Check sheet for the modelled part. Datum: model origin and axes. Units: mm. A direction names the side the tool comes from. Round coordinates to 2 decimals unless told otherwise and drop trailing zeros. Loops run counter-clockwise (first coordinate to the right, second up) from the corner with the lowest first, then second, coordinate; pieces in that order, holes last. Notation, with made-up numbers: M 67.5,-5.5 L 97.5,-5.5 A17 ccw 97.5,27.5 Z; hole C 39,-36.5 d1. An arc over 180 degrees is marked long. Write item = value, one per line. Start each with the question number.
(1) Set-up check for faces 1 (the face through (-38, -3, -9.525)), 2 (the face through (76.2, -3, -1)): record each of +Z, -Z, +X, -X, +Y, -Y from which the full face is reachable in a straight line by a thin tool's end or side.
(2) Go/stop test with flat-tipped pins: P1, Ø8, axis at x = 36.5, z = 8.5, coming from the +Y side; P2, Ø11.5, axis at x = 38.1, z = -30.48, coming from the +Y side. Record where each tip stops, or that it passes through.
(3) Mould release check, pull along Z, two halves, no side actions. Record for faces 3 (the face through (-72.58, -3.22, -53.33)), 4 (the face through (72.58, -3.22, 53.33)), 5 (the face through (-38, -3, -3.175)): pulls with the +Z half, pulls with the -Z half, needs draft (parallel to the pull), parting line crosses it, or undercut.
(4) Cross-section at A-A on x = 38.1. Record the boundary of the cut face in (y, z) (3 decimals).
(5) Scan lines: L1, parallel to Z at x = 38.1, y = -4 (3 decimals); L2, parallel to Z at x = 33, y = -3.75; L3, parallel to X at y = -4.25, z = 29. Record each from-to range of solid material in increasing order. Write a range as from..to.
(6) Cross-section at C-C on x = -27.5. State how many separate pieces and enclosed holes the cut face has, plus the area to 3 significant figures.
(7) Cross-section at B-B on z = 0. Record the boundary of the cut face in (x, y) (3 decimals), plus the area to 3 significant figures.
from build123d import *

# Parameters (mm, degrees)
F0_W         = 152.4
F0_H         = 114.3
F1_DEPTH     = 6.35
F2_R         = 12.7
F3_R         = 9.525
F4_DEPTH     = 25.4
F5_R         = 9.525
F6_DEPTH     = 25.4
F7_R         = 9.525
F8_DEPTH     = 25.4
F16_W        = 50.8
F16_H        = 6.35
F15_W        = 50.8
F15_H        = 6.35
F14_W        = 50.8
F14_H        = 6.35
F13_W        = 50.8
F13_H        = 6.35
F12_W        = 50.8
F12_H        = 6.35
F11_W        = 50.8
F11_H        = 6.35
F10_W        = 50.8
F10_H        = 6.35
F9_W         = 50.8
F9_H         = 6.35
F17_DEPTH    = 25.4
F18_T1_DEPTH = 6.35
F19_T1_DEPTH = 6.35


# Not quite as in the source:
# - a fillet or chamfer that OpenCascade refuses, or shapes differently, is made with other operations: its cross-section is extruded or revolved along the edge and cut away or added


with BuildPart() as f1:
    # F0 (on Front) → F1 (new body)
    with BuildSketch(Plane.XZ):
        Rectangle(F0_W, F0_H)
    extrude(amount=F1_DEPTH)

    # F2
    f2_edges = [f1.edges().sort_by_distance(p)[0] for p in [
        (-76.2, -3.175, 57.15),
        (-76.2, -3.175, -57.15),
        (76.2, -3.175, -57.15),
        (76.2, -3.175, 57.15),
    ]]
    fillet(f2_edges, radius=F2_R)

    # F3 (on face) → F4 (cut)
    with BuildSketch(Plane.XZ.offset(6.35)):
        with Locations((38.1, 30.48)):
            Circle(F3_R)
    extrude(amount=-F4_DEPTH, mode=Mode.SUBTRACT)

    # F5 (on face) → F6 (cut)
    with BuildSketch(Plane.XZ.offset(6.35)):
        with Locations((38.1, 0)):
            Circle(F5_R)
    extrude(amount=-F6_DEPTH, mode=Mode.SUBTRACT)

    # F7 (on face) → F8 (cut)
    with BuildSketch(Plane.XZ.offset(6.35)):
        with Locations((38.1, -30.48)):
            Circle(F7_R)
    extrude(amount=-F8_DEPTH, mode=Mode.SUBTRACT)

    # F16 (on face) + F15 (on face) + F14 (on face) + F13 (on face) + F12 (on face) + F11 (on face) + F10 (on face) + F9 (on face) → F17 (cut)
    with BuildSketch(Plane.XZ.offset(6.35)):
        with Locations((-38.1, 44.45)):
            Rectangle(F16_W, F16_H)
    with BuildSketch(Plane.XZ.offset(6.35)):
        with Locations((-38.1, 31.75)):
            Rectangle(F15_W, F15_H)
    with BuildSketch(Plane.XZ.offset(6.35)):
        with Locations((-38.1, 19.05)):
            Rectangle(F14_W, F14_H)
    with BuildSketch(Plane.XZ.offset(6.35)):
        with Locations((-38.1, 6.35)):
            Rectangle(F13_W, F13_H)
    with BuildSketch(Plane.XZ.offset(6.35)):
        with Locations((-38.1, -6.35)):
            Rectangle(F12_W, F12_H)
    with BuildSketch(Plane.XZ.offset(6.35)):
        with Locations((-38.1, -19.05)):
            Rectangle(F11_W, F11_H)
    with BuildSketch(Plane.XZ.offset(6.35)):
        with Locations((-38.1, -31.75)):
            Rectangle(F10_W, F10_H)
    with BuildSketch(Plane.XZ.offset(6.35)):
        with Locations((-38.1, -44.45)):
            Rectangle(F9_W, F9_H)
    extrude(amount=-F17_DEPTH, mode=Mode.SUBTRACT)

    # F18: fillet of radius 3.81 on 16 edges, made by hand

    # F18_s2 → F18_t1 (join)
    with BuildSketch(Plane.XZ):
        with BuildLine():
            ThreePointArc((-12.7, 6.985), (-13.8159231637, 4.2909231637), (-16.51, 3.175))
            Line((-16.51, 3.175), (-12.7, 3.175))
            Line((-12.7, 3.175), (-12.7, 6.985))
        make_face()
        with BuildLine():
            ThreePointArc((-16.51, -9.525), (-13.8159231637, -8.4090768363), (-12.7, -5.715))
            Line((-12.7, -5.715), (-12.7, -9.525))
            Line((-12.7, -9.525), (-16.51, -9.525))
        make_face()
        with BuildLine():
            ThreePointArc((-12.7, -31.115), (-13.8159231637, -33.8090768363), (-16.51, -34.925))
            Line((-16.51, -34.925), (-12.7, -34.925))
            Line((-12.7, -34.925), (-12.7, -31.115))
        make_face()
        with BuildLine():
            ThreePointArc((-16.51, -22.225), (-13.8159231637, -21.1090768363), (-12.7, -18.415))
            Line((-12.7, -18.415), (-12.7, -22.225))
            Line((-12.7, -22.225), (-16.51, -22.225))
        make_face()
        with BuildLine():
            ThreePointArc((-12.7, -43.815), (-13.8159231637, -46.5090768363), (-16.51, -47.625))
            Line((-16.51, -47.625), (-12.7, -47.625))
            Line((-12.7, -47.625), (-12.7, -43.815))
        make_face()
        with BuildLine():
            ThreePointArc((-16.51, 15.875), (-13.8159231637, 16.9909231637), (-12.7, 19.685))
            Line((-12.7, 19.685), (-12.7, 15.875))
            Line((-12.7, 15.875), (-16.51, 15.875))
        make_face()
        with BuildLine():
            ThreePointArc((-16.51, 28.575), (-13.8159231637, 29.6909231637), (-12.7, 32.385))
            Line((-12.7, 32.385), (-12.7, 28.575))
            Line((-12.7, 28.575), (-16.51, 28.575))
        make_face()
        with BuildLine():
            ThreePointArc((-16.51, 41.275), (-13.8159231637, 42.3909231637), (-12.7, 45.085))
            Line((-12.7, 45.085), (-12.7, 41.275))
            Line((-12.7, 41.275), (-16.51, 41.275))
        make_face()
        with BuildLine():
            ThreePointArc((-12.7, -45.085), (-13.8159231637, -42.3909231637), (-16.51, -41.275))
            Line((-16.51, -41.275), (-12.7, -41.275))
            Line((-12.7, -41.275), (-12.7, -45.085))
        make_face()
        with BuildLine():
            ThreePointArc((-12.7, -32.385), (-13.8159231637, -29.6909231637), (-16.51, -28.575))
            Line((-16.51, -28.575), (-12.7, -28.575))
            Line((-12.7, -28.575), (-12.7, -32.385))
        make_face()
        with BuildLine():
            ThreePointArc((-12.7, -19.685), (-13.8159231637, -16.9909231637), (-16.51, -15.875))
            Line((-16.51, -15.875), (-12.7, -15.875))
            Line((-12.7, -15.875), (-12.7, -19.685))
        make_face()
        with BuildLine():
            ThreePointArc((-12.7, -6.985), (-13.8159231637, -4.2909231637), (-16.51, -3.175))
            Line((-16.51, -3.175), (-12.7, -3.175))
            Line((-12.7, -3.175), (-12.7, -6.985))
        make_face()
        with BuildLine():
            ThreePointArc((-12.7, 5.715), (-13.8159231637, 8.4090768363), (-16.51, 9.525))
            Line((-16.51, 9.525), (-12.7, 9.525))
            Line((-12.7, 9.525), (-12.7, 5.715))
        make_face()
        with BuildLine():
            ThreePointArc((-12.7, 18.415), (-13.8159231637, 21.1090768363), (-16.51, 22.225))
            Line((-16.51, 22.225), (-12.7, 22.225))
            Line((-12.7, 22.225), (-12.7, 18.415))
        make_face()
        with BuildLine():
            ThreePointArc((-12.7, 31.115), (-13.8159231637, 33.8090768363), (-16.51, 34.925))
            Line((-16.51, 34.925), (-12.7, 34.925))
            Line((-12.7, 34.925), (-12.7, 31.115))
        make_face()
        with BuildLine():
            ThreePointArc((-12.7, 43.815), (-13.8159231637, 46.5090768363), (-16.51, 47.625))
            Line((-16.51, 47.625), (-12.7, 47.625))
            Line((-12.7, 47.625), (-12.7, 43.815))
        make_face()
    extrude(amount=F18_T1_DEPTH)

    # F19: fillet of radius 3.81 on 16 edges, made by hand

    # F19_s2 → F19_t1 (join)
    with BuildSketch(Plane.XZ):
        with BuildLine():
            ThreePointArc((-59.69, 47.625), (-62.3840768363, 46.5090768363), (-63.5, 43.815))
            Line((-63.5, 43.815), (-63.5, 47.625))
            Line((-63.5, 47.625), (-59.69, 47.625))
        make_face()
        with BuildLine():
            ThreePointArc((-59.69, 34.925), (-62.3840768363, 33.8090768363), (-63.5, 31.115))
            Line((-63.5, 31.115), (-63.5, 34.925))
            Line((-63.5, 34.925), (-59.69, 34.925))
        make_face()
        with BuildLine():
            ThreePointArc((-59.69, 22.225), (-62.3840768363, 21.1090768363), (-63.5, 18.415))
            Line((-63.5, 18.415), (-63.5, 22.225))
            Line((-63.5, 22.225), (-59.69, 22.225))
        make_face()
        with BuildLine():
            ThreePointArc((-59.69, 9.525), (-62.3840768363, 8.4090768363), (-63.5, 5.715))
            Line((-63.5, 5.715), (-63.5, 9.525))
            Line((-63.5, 9.525), (-59.69, 9.525))
        make_face()
        with BuildLine():
            ThreePointArc((-59.69, -3.175), (-62.3840768363, -4.2909231637), (-63.5, -6.985))
            Line((-63.5, -6.985), (-63.5, -3.175))
            Line((-63.5, -3.175), (-59.69, -3.175))
        make_face()
        with BuildLine():
            ThreePointArc((-59.69, -15.875), (-62.3840768363, -16.9909231637), (-63.5, -19.685))
            Line((-63.5, -19.685), (-63.5, -15.875))
            Line((-63.5, -15.875), (-59.69, -15.875))
        make_face()
        with BuildLine():
            ThreePointArc((-59.69, -28.575), (-62.3840768363, -29.6909231637), (-63.5, -32.385))
            Line((-63.5, -32.385), (-63.5, -28.575))
            Line((-63.5, -28.575), (-59.69, -28.575))
        make_face()
        with BuildLine():
            ThreePointArc((-59.69, -41.275), (-62.3840768363, -42.3909231637), (-63.5, -45.085))
            Line((-63.5, -45.085), (-63.5, -41.275))
            Line((-63.5, -41.275), (-59.69, -41.275))
        make_face()
        with BuildLine():
            ThreePointArc((-59.69, 41.275), (-62.3840768363, 42.3909231637), (-63.5, 45.085))
            Line((-63.5, 45.085), (-63.5, 41.275))
            Line((-63.5, 41.275), (-59.69, 41.275))
        make_face()
        with BuildLine():
            ThreePointArc((-59.69, 28.575), (-62.3840768363, 29.6909231637), (-63.5, 32.385))
            Line((-63.5, 32.385), (-63.5, 28.575))
            Line((-63.5, 28.575), (-59.69, 28.575))
        make_face()
        with BuildLine():
            ThreePointArc((-59.69, 15.875), (-62.3840768363, 16.9909231637), (-63.5, 19.685))
            Line((-63.5, 19.685), (-63.5, 15.875))
            Line((-63.5, 15.875), (-59.69, 15.875))
        make_face()
        with BuildLine():
            ThreePointArc((-63.5, 6.985), (-62.3840768363, 4.2909231637), (-59.69, 3.175))
            Line((-59.69, 3.175), (-63.5, 3.175))
            Line((-63.5, 3.175), (-63.5, 6.985))
        make_face()
        with BuildLine():
            ThreePointArc((-59.69, -9.525), (-62.3840768363, -8.4090768363), (-63.5, -5.715))
            Line((-63.5, -5.715), (-63.5, -9.525))
            Line((-63.5, -9.525), (-59.69, -9.525))
        make_face()
        with BuildLine():
            ThreePointArc((-59.69, -22.225), (-62.3840768363, -21.1090768363), (-63.5, -18.415))
            Line((-63.5, -18.415), (-63.5, -22.225))
            Line((-63.5, -22.225), (-59.69, -22.225))
        make_face()
        with BuildLine():
            ThreePointArc((-63.5, -31.115), (-62.3840768363, -33.8090768363), (-59.69, -34.925))
            Line((-59.69, -34.925), (-63.5, -34.925))
            Line((-63.5, -34.925), (-63.5, -31.115))
        make_face()
        with BuildLine():
            ThreePointArc((-63.5, -43.815), (-62.3840768363, -46.5090768363), (-59.69, -47.625))
            Line((-59.69, -47.625), (-63.5, -47.625))
            Line((-63.5, -47.625), (-63.5, -43.815))
        make_face()
    extrude(amount=F19_T1_DEPTH)


solid = f1.part
Result:
q1.face_1 = +Y, -Y
q1.face_2 = +Z, -Z, +X, +Y, -Y
q2.P1 = 0
q2.P2 = through
q3.face_3 = pulls with the -Z half
q3.face_4 = pulls with the +Z half
q3.face_5 = undercut
q4.outline = M -6.35,-57.15 L 0,-57.15 L 0,-40.005 L -6.35,-40.005 Z; M -6.35,-20.955 L 0,-20.955 L 0,-9.525 L -6.35,-9.525 Z; M -6.35,9.525 L 0,9.525 L 0,20.955 L -6.35,20.955 Z; M -6.35,40.005 L 0,40.005 L 0,57.15 L -6.35,57.15 Z
q5.L1 = -57.15..-40.005, -20.955..-9.525, 9.525..20.955, 40.005..57.15
q5.L2 = -57.15..-38.52, -22.44..-8.04, 8.04..22.44, 38.52..57.15
q5.L3 = -76.2..-61.44, -14.76..28.69, 47.51..76.2
q6.separate_pieces = 9
q6.enclosed_holes = 0
q6.area = 403 mm^2
q7.outline = M -76.2,-6.35 L 28.575,-6.35 L 28.575,0 L -76.2,0 Z; M 47.625,-6.35 L 76.2,-6.35 L 76.2,0 L 47.625,0 Z
q7.area = 847 mm^2
